Source: CAD feature listing. Evaluate the final solid. Frame: model axes, mm. Face numbers are marked on the shaded views. Give positions to 0.01 mm unless a question says otherwise; leave off trailing zeros. Loops run counter-clockwise (first coordinate to the right, second up) from the corner with the lowest first, then second, coordinate; pieces in that order, holes last.
from build123d import *

# Parameters (mm, degrees)
SKETCH1_R               = 88.265
BOSS_EXTRUDE1_DEPTH     = 25.4
SKETCH2_R               = 76.2
CUT_EXTRUDE1_DEPTH      = 8.89
SKETCH3_R               = 70.231
CUT_EXTRUDE2_DEPTH      = 3.175
SKETCH4_R               = 66.675
CUT_EXTRUDE3_DEPTH      = 126.535822278
CHAMFER1_SIZE           = 10.16
CHAMFER1_SIZE2          = 18.415
CHAMFER2_SIZE           = 20.32
CHAMFER2_SIZE2          = 5.08
CUT_EXTRUDE4_DEPTH      = 128.383595686
CUT_EXTRUDE4_DEPTH_BACK = 128.383595686
SKETCH5_R               = 1.35255


with BuildPart() as part:
    # Sketch1 → Boss-Extrude1 (new body)
    with BuildSketch(Plane.XY):
        Circle(SKETCH1_R)
    extrude(amount=BOSS_EXTRUDE1_DEPTH)

    # Sketch2 → Cut-Extrude1 (cut)
    with BuildSketch(Plane.XY.offset(25.4)):
        Circle(SKETCH2_R)
    extrude(amount=-CUT_EXTRUDE1_DEPTH, mode=Mode.SUBTRACT)

    # Sketch3 → Cut-Extrude2 (cut)
    with BuildSketch(Plane.XY.offset(16.51)):
        Circle(SKETCH3_R)
    extrude(amount=-CUT_EXTRUDE2_DEPTH, mode=Mode.SUBTRACT)

    # Sketch4 → Cut-Extrude3 (cut, through all)
    with BuildSketch(Plane.XY.offset(13.335)):
        Circle(SKETCH4_R)
    extrude(amount=-CUT_EXTRUDE3_DEPTH, mode=Mode.SUBTRACT)

    # Chamfer1
    chamfer1_edges = [part.edges().sort_by_distance(p)[0] for p in [
        (-66.675, 0, 0),
    ]]
    chamfer1_side = [part.faces().sort_by_distance(p)[0] for p in [
        (-66.675, 0, 6.6675),
    ]]
    chamfer(chamfer1_edges, length=CHAMFER1_SIZE, length2=CHAMFER1_SIZE2, reference=chamfer1_side[0])

    # Chamfer2
    chamfer2_edges = [part.edges().sort_by_distance(p)[0] for p in [
        (-88.265, 0, 25.4),
    ]]
    chamfer2_side = [part.faces().sort_by_distance(p)[0] for p in [
        (-88.265, 0, 12.7),
    ]]
    chamfer(chamfer2_edges, length=CHAMFER2_SIZE, length2=CHAMFER2_SIZE2, reference=chamfer2_side[0])

    # Sketch5 → Cut-Extrude4 (cut, two sides: drawn at the far end of the back side and taken through both)
    with BuildSketch(Plane(origin=(0, 0, 0), x_dir=(1, 0, 0), z_dir=(0, 1, 0)).offset(-CUT_EXTRUDE4_DEPTH_BACK)):
        with Locations(Location((0, -21.59, 0), (0, 0, 270))):
            Circle(SKETCH5_R)
    extrude(amount=CUT_EXTRUDE4_DEPTH + CUT_EXTRUDE4_DEPTH_BACK, mode=Mode.SUBTRACT)


solid = part.part
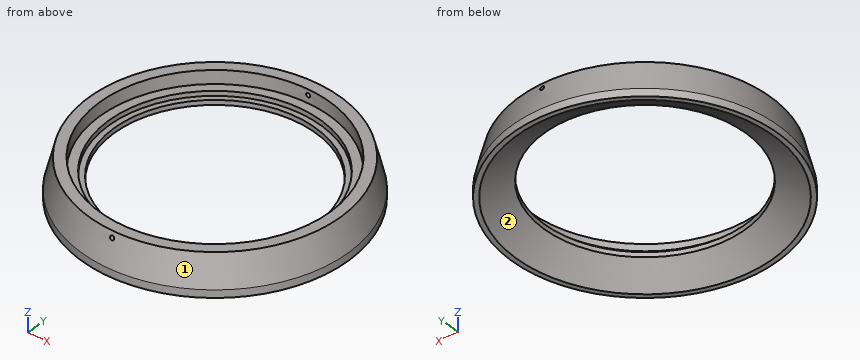
1) Cut plane A-A (y = 0). Return loops of the section in (x, z) (3 decimals).
Checks:
outline: (-88.265, 0) - (-85.09, 0) - (-66.675, 10.16) - (-66.675, 13.335) - (-70.231, 13.335) - (-70.231, 16.51) - (-76.2, 16.51) - (-76.2, 25.4) - (-83.185, 25.4) - (-88.265, 5.08) - close; (66.675, 10.16) - (85.09, 0) - (88.265, 0) - (88.265, 5.08) - (83.185, 25.4) - (76.2, 25.4) - (76.2, 16.51) - (70.231, 16.51) - (70.231, 13.335) - (66.675, 13.335) - close
2) Pull-direction query (X, two-part tool) for the marked faces 1 and 2; classes: released by +X, released by -X, zero draft, split by the parting line, or undercut.
Checks:
face 1: split by the parting line
face 2: undercut
3) Ray query, probe 1 along X at (y, z) = (-21.5, 6.5); probe 2 along Y at (x, z) = (45.5, 9); probe 3 along X at (y, z) = (44, 24.25). Return the intervals inside material, ascending.
Checks:
probe 1: x = -85.24 to -70.09, 70.09 to 85.24
probe 2: y = -74.49 to -51.58, 51.58 to 74.49
probe 3: x = -70.93 to -62.21, 62.21 to 70.93
4) Contact query for flat-ended pins moving along their axis: P1, Ø1.5, axis at x = 38, z = 21.5, coming from the +Y side; P2, Ø10, axis at x = -24.5, z = 9, coming from the -Y side; P3, Ø1.5, axis at x = 35, z = 15, coming from the -Y side. Output: stop coordinate, or through.
Checks:
P1: stops at y = 75.52
P2: stops at y = -85.64
P3: stops at y = -78.71
